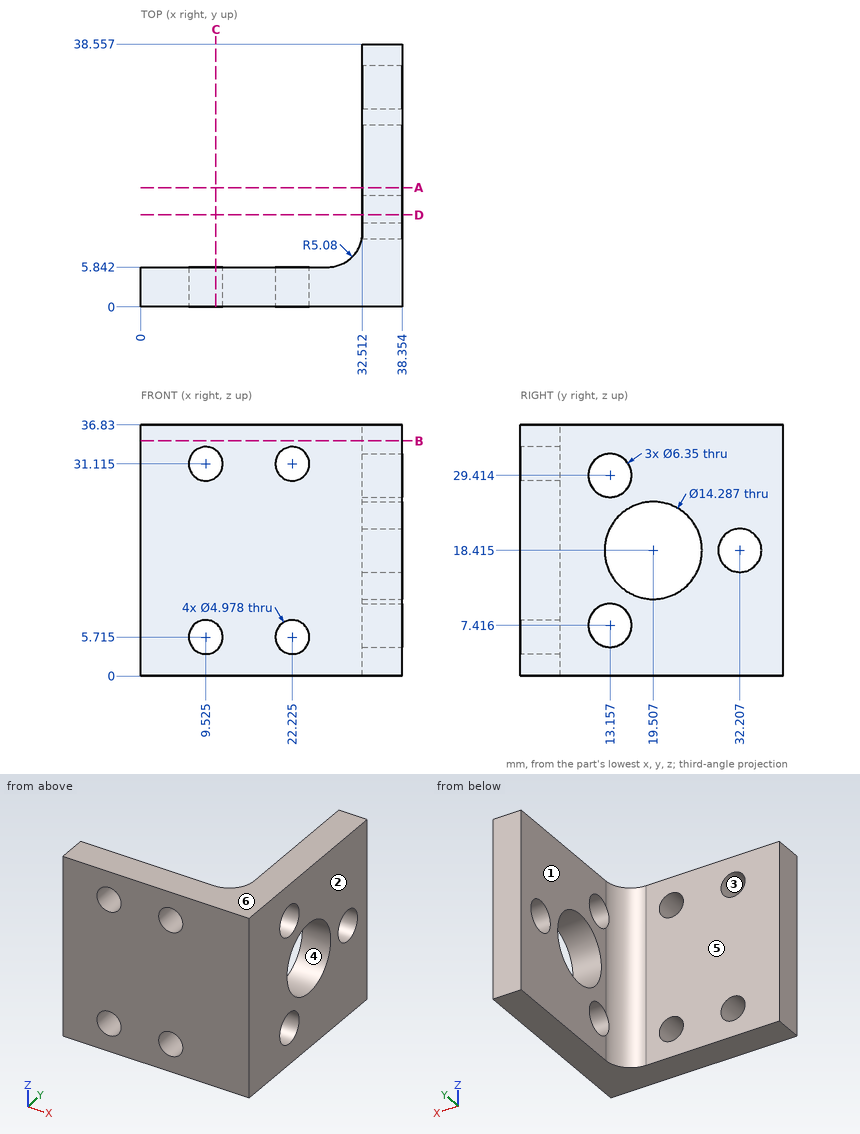
Input: dimensioned drawing with shaded views. Units: mm. Origin: part minimum x, y, z. A direction names the side the tool comes from. Give positions to 0.01 mm unless a question says otherwise; leave off trailing zeros. Order: outer loops, then holes, each group sorted by start corner. A loop starts at its lowest first (then second) coordinate and runs counter-clockwise, first axis right, second up. Notation, with made-up numbers: (-36, 30) -> (21, 30) arc R11 ccw to (21, 47) -> close; hole circle Ø11 at (46, 80.25). An arc over 180 degrees is marked (long way). Answer as a JSON object with one key per item and string values.
Q1. Section B-B (z = 34.5). Output: boundary loops of the cut face in (x, y) (1 decimal).
Entries:
{"outline": "(0, 0) -> (38.4, 0) -> (38.4, 38.6) -> (32.5, 38.6) -> (32.5, 10.9) arc R5.1 cw to (27.4, 5.8) -> (0, 5.8) -> close"}
Q2. First-contact query: pin 1 (8.5 mm diameter, centred on y = 13.16, z = 7.42, fed in from -X); pin 2 (6 mm diameter, centred on x = 16.5, z = 25, fed in from +Y); pin 3 (8.5 mm diameter, centred on y = 23.5, z = 16.5, fed in from -X). Flat tips, straight axial feed; report the tip coordinate or a pass-through.
Entries:
{"pin 1": "stops at x = 32.1", "pin 2": "stops at y = 5.84", "pin 3": "stops at x = 32.51"}
Q3. Draft query along Z for the marked faces 3, 4, 5 and 6. Return one class per face: released by +Z, released by -Z, zero draft, split by the parting line, or undercut.
Entries:
{"face 3": "undercut", "face 4": "undercut", "face 5": "zero draft", "face 6": "released by +Z"}
Q4. Access query for the marked faces 1 and 2. Directions: +Z, -Z, +X, -X, +Y, -Y. A direction counts if a zero-diameter tool reaches every point of the face in a straight line with its end or side. Return the directions, or none.
Entries:
{"face 1": "+Z, -Z, -X, +Y", "face 2": "+Z, -Z, +X, +Y, -Y"}
Q5. Material intervals for probe 1 along X at (y, z) = (31.5, 28.5) (1 decimal); probe 2 along Y at (x, z) = (15, 28.5); probe 3 along Z at (x, y) = (9, 2), sorted ascending.
Entries:
{"probe 1": "x = 32.5 to 38.4", "probe 2": "y = 0 to 5.84", "probe 3": "z = 0 to 3.28, 8.15 to 28.68, 33.55 to 36.83"}
Q6. Section C-C (x = 11). Output: boundary loops of the cut face in (y, z).
Entries:
{"outline": "(0, 0) -> (5.84, 0) -> (5.84, 3.71) -> (0, 3.71) -> close; (0, 7.72) -> (5.84, 7.72) -> (5.84, 29.11) -> (0, 29.11) -> close; (0, 33.12) -> (5.84, 33.12) -> (5.84, 36.83) -> (0, 36.83) -> close"}
Q7. Section A-A (y = 17.5). Output: boundary loops of the cut face in (x, z) (1 decimal), plus the area to 3 significant figures.
Entries:
{"outline": "(32.5, 0) -> (38.4, 0) -> (38.4, 11.6) -> (32.5, 11.6) -> close; (32.5, 25.3) -> (38.4, 25.3) -> (38.4, 36.8) -> (32.5, 36.8) -> close", "area": "135 mm^2"}
Q8. Section D-D (y = 13.5). Output: boundary loops of the cut face in (x, z) (1 decimal).
Entries:
{"outline": "(32.5, 0) -> (38.4, 0) -> (38.4, 4.3) -> (32.5, 4.3) -> close; (32.5, 10.6) -> (38.4, 10.6) -> (38.4, 14.5) -> (32.5, 14.5) -> close; (32.5, 22.3) -> (38.4, 22.3) -> (38.4, 26.3) -> (32.5, 26.3) -> close; (32.5, 32.6) -> (38.4, 32.6) -> (38.4, 36.8) -> (32.5, 36.8) -> close"}
